The drawing under review shows one solid part. Ordinate dimensions are in mm from its lowest x, y, z. A direction names the side the tool comes from. Coordinates: 2 decimals unless noted, no trailing zeros. Order: outer loops, then holes, each group sorted by start corner. A loop starts at its lowest first (then second) coordinate and runs counter-clockwise, first axis right, second up.
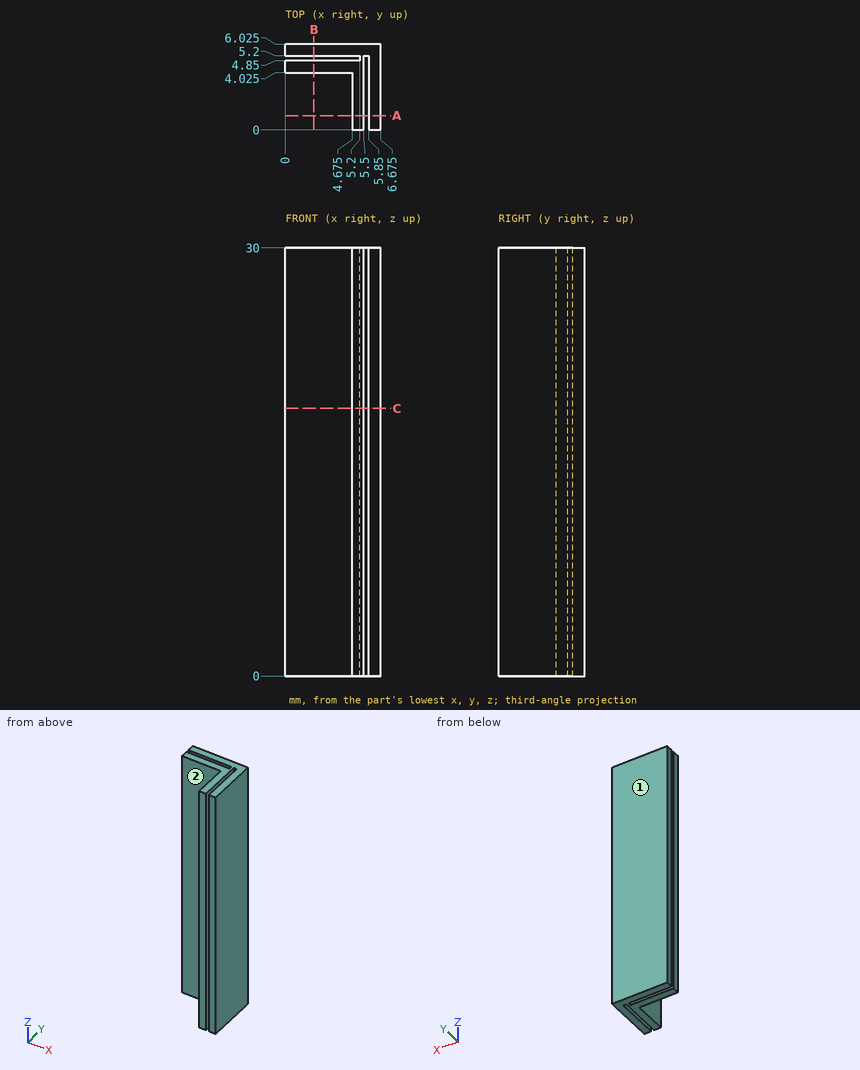
1. Machinability: for the marked faces 1 and 2, which of the approach directions +Z, -Z, +X, -X, +Y, -Y give a long, thin tool a straight path to every point of the face, cutting with its end or side? Answer none if there is none.
Answer below:
face 1: +Z, -Z, +X, -X, +Y
face 2: +Z, -Z, -X, -Y
2. Take a section at C-C, the plane z = 18.75. Give the boundary of the cut face in (x, y) (3 decimals).
Answer below:
outline: (0, 4.025) - (4.675, 4.025) - (4.675, 0) - (5.5, 0) - (5.5, 5.2) - (5.85, 5.2) - (5.85, 0) - (6.675, 0) - (6.675, 6.025) - (0, 6.025) - (0, 5.2) - (5.2, 5.2) - (5.2, 4.85) - (0, 4.85) - close
3. Clearance check with flat-ended pins moving along their axes: pin 1 Ø2 at (x, z) = (4.5, 3.5) entering from -Y; pin 2 Ø3 at (y, z) = (1.5, 20.5) entering from -X (3 decimals); pin 3 Ø1.4 at (x, z) = (3, 17.5) entering from -Y (3 decimals). State where each tip first meets the part, or that it passes through.
Answer below:
pin 1: stops at y = 0
pin 2: stops at x = 4.675
pin 3: stops at y = 4.025
4. To check wall thickness, follow L1, parallel to X at y = 4.5, z = 4.5 (3 decimals); L2, parallel to X at y = 0.5, z = 4.25 (3 decimals); L3, parallel to Y at x = 3.5, z = 5.5 (3 decimals). State the ranges of each line that lie inside material, in increasing order.
Answer below:
L1: x = 0 to 5.5, 5.85 to 6.675
L2: x = 4.675 to 5.5, 5.85 to 6.675
L3: y = 4.025 to 4.85, 5.2 to 6.025
5. Take a section at A-A, the plane y = 1. Give the boundary of the cut face in (x, z) (3 decimals), plus the area to 3 significant figures.
Answer below:
outline: (4.675, 0) - (5.5, 0) - (5.5, 30) - (4.675, 30) - close; (5.85, 0) - (6.675, 0) - (6.675, 30) - (5.85, 30) - close
area: 49.5 mm2
6. Take a section at B-B, the plane x = 2. Give the boundary of the cut face in (y, z) (3 decimals), plus the area to 3 significant figures.
Answer below:
outline: (4.025, 0) - (4.85, 0) - (4.85, 30) - (4.025, 30) - close; (5.2, 0) - (6.025, 0) - (6.025, 30) - (5.2, 30) - close
area: 49.5 mm2
